Could you check a few things on this model? Use its own coordinates, in mm. Round coordinates to 2 decimals unless told otherwise and drop trailing zeros. Loops run counter-clockwise (first coordinate to the right, second up) from the corner with the lowest first, then second, coordinate; pieces in that order, holes last. Notation, with made-up numbers: M 44,-27.5 L 97,-27.5 A16 cw 97,1.5 Z; hole C 52,-31 d8. An arc over 180 degrees is marked long. Answer in a Markdown table with one row per item.
```python
from build123d import *

# Parameters (mm, degrees)
SKETCH1_W           = 8
SKETCH1_H           = 8
BOSS_EXTRUDE1_DEPTH = 14.05
SKETCH2_R           = 1.75
CUT_EXTRUDE1_DEPTH  = 16.308633478
SKETCH3_W           = 14.05
SKETCH3_H           = 8
BOSS_EXTRUDE2_DEPTH = 10
SKETCH4_R           = 1.75
CUT_EXTRUDE2_DEPTH  = 22.586444055


with BuildPart() as part:
    # Sketch1 → Boss-Extrude1 (new body)
    with BuildSketch(Plane.XY):
        with Locations((0.302869186, -0.293841606)):
            Rectangle(SKETCH1_W, SKETCH1_H)
    extrude(amount=BOSS_EXTRUDE1_DEPTH)

    # Sketch2 → Cut-Extrude1 (cut, through all)
    with BuildSketch(Plane.XY.offset(14.05)):
        with Locations((0.302869186, -0.293841606)):
            Circle(SKETCH2_R)
    extrude(amount=-CUT_EXTRUDE1_DEPTH, mode=Mode.SUBTRACT)

    # Sketch3 → Boss-Extrude2 (add)
    with BuildSketch(Plane(origin=(4.302869186, 0, 0), x_dir=(0, 0, -1), z_dir=(1, 0, 0))):
        with Locations((-7.025, -0.293841606)):
            Rectangle(SKETCH3_W, SKETCH3_H)
    extrude(amount=BOSS_EXTRUDE2_DEPTH)

    # Sketch4 → Cut-Extrude2 (cut, through all)
    with BuildSketch(Plane(origin=(0, 3.706158394, 0), x_dir=(1, 0, 0), z_dir=(0, 1, 0))):
        with Locations(Location((8.302869186, -7.025, 0), (0, 0, 270))):
            Circle(SKETCH4_R)
    extrude(amount=-CUT_EXTRUDE2_DEPTH, mode=Mode.SUBTRACT)


solid = part.part
```
1) I want a section at C-C, the plane z = 5.75. Please give me the cut outline in (x, y), plus the area to 3 significant figures.
Computed:
| item | result |
|---|---|
| outline | M -3.7,-4.29 L 7.1,-4.29 L 7.1,3.71 L -3.7,3.71 Z; M 9.5,-4.29 L 14.3,-4.29 L 14.3,3.71 L 9.5,3.71 Z; hole C 0.3,-0.29 d3.5 |
| area | 115 mm² |
2) I need wall thicknesses on line 1 (X direction, y = -2.75, z = 7); line 2 (X direction, y = -1.75, z = 6.75); line 3 (X direction, y = -1, z = 5.75). Which ranges of each line are inside material? Lowest first, please.
Computed:
| item | result |
|---|---|
| line 1 | x = -3.7 to 6.55, 10.05 to 14.3 |
| line 2 | x = -3.7 to -0.67, 1.27 to 6.57, 10.03 to 14.3 |
| line 3 | x = -3.7 to -1.3, 1.9 to 7.1, 9.5 to 14.3 |
3) I want a section at D-D, the plane y = 3.25. Please give me the cut outline in (x, z) (3 decimals).
Computed:
| item | result |
|---|---|
| outline | M -3.697,0 L 14.303,0 L 14.303,14.05 L -3.697,14.05 Z; hole C 8.303,7.025 d3.5 |
4) If we mould it in two halves opening along X, with no side actions, what happens to faces 1 (the face through (0.08, 1.44, 7.12)), 2 (the face through (5, -4.294, 7)), 3 (the face through (9.778, -0.238, 7.966)), 4 (the face through (-3.697, 0, 7))? For each: released by +X, released by -X, zero draft, split by the parting line, or undercut.
Computed:
| item | result |
|---|---|
| face 1 | undercut |
| face 2 | zero draft |
| face 3 | undercut |
| face 4 | released by -X |
5) I want a section at A-A, the plane y = 1.25. Please give me the cut outline in (x, z) (3 decimals).
Computed:
| item | result |
|---|---|
| outline | M -3.697,0 L -0.521,0 L -0.521,14.05 L -3.697,14.05 Z; M 1.127,0 L 14.303,0 L 14.303,14.05 L 1.127,14.05 Z; hole C 8.303,7.025 d3.5 |
6) I want a section at B-B, the plane x = -1. Please give me the cut outline in (y, z), plus the area to 3 significant figures.
Computed:
| item | result |
|---|---|
| outline | M -4.29,0 L -1.46,0 L -1.46,14.05 L -4.29,14.05 Z; M 0.87,0 L 3.71,0 L 3.71,14.05 L 0.87,14.05 Z |
| area | 79.6 mm² |
7) Will this pin go through, and if not, where does the flat tip stop? P1, Ø4.5, axis at x = 0.3, y = -0.29, coming from the +Z side.
Computed:
| item | result |
|---|---|
| P1 | stops at z = 14.05 |
